The model under review builds one solid part; all positions refer to its coordinate system, in mm. A direction names the side the tool comes from. Round coordinates to 2 decimals unless told otherwise and drop trailing zeros. Write each loop counter-clockwise with the first axis right and the second up, starting at its lowest first coordinate (ties: lowest second). Pieces come first, ordered by that corner, then holes. Notation, with made-up numbers: (18, 17.5) -> (42, 17.5) arc R25 ccw to (42, 43.5) -> close; hole circle Ø5 at (5, 67.25). An arc over 180 degrees is marked (long way). Answer as a JSON object with one key per item and string values. Group by question number.
1) Machinability: for faces 5 (the flat face through (0, -20, 0)), 6 (the cylindrical face through (-50, -5, 0)), which of the approach directions +Z, -Z, +X, -X, +Y, -Y give a long, thin tool a straight path to every point of the face, cutting with its end or side? Answer none if there is none.
2) We need section B-B, the plane x = 0. Write out the cut boundary in (y, z), then the cut area to 3 significant figures.
3) We need section A-A, the plane y = -8.75. Write out the cut boundary in (x, z).
4) Mouldability with a two-part tool opening along X and no side actions: class faces 1 (the flat face through (23.664, -4.93, 14.526)), 2 (the flat face through (27, -10, 0)), 3 (the flat face through (-23.664, -4.93, -14.526)), 4 (the cylindrical face through (35, -5, 0)) as pulls with the +X half, pulls with the -X half, needs draft (parallel to the pull), parting line crosses it, or undercut.
5) To check wall thickness, follow probe 1 along Y at (x, z) = (-27, -7); probe 2 along Z at (x, y) = (40, -4); probe 3 along Z at (x, y) = (13.5, -26). State the ranges of each line that lie inside material, in increasing order. Write a range as [from, to].
6) We need section C-C, the plane x = -43. Write out the cut boundary in (y, z), then the cut area to 3 significant figures.
7) Insertion check: pin 1 Ø1 at (y, z) = (-15.5, -4.5) entering from -X; pin 2 Ø15 at (x, z) = (-5.5, -4.5) entering from -Y; pin 3 Ø3 at (x, z) = (-32.5, -7.5) entering from -Y; pin 4 Ø8 at (x, z) = (40, 0) entering from +Y. Each pin has a flat end and moves straight along its axis. Give the tip position at first contact, or say it passes through.
from build123d import *

# Parameters (mm, degrees)
F1_DEPTH = 10
F2_R     = 5
F3_DEPTH = 10.001
F5_DEPTH = 20
F6_R     = 15
F7_DEPTH = 10


with BuildPart() as f1:
    # F0 (on Front) → F1 (new body)
    with BuildSketch(Plane.XZ):
        with BuildLine():
            Line((5.158226, -19.323372), (41.659475, -9.861346))
            ThreePointArc((41.659475, -9.861346), (50, 0), (41.659475, 9.861346))
            Line((41.659475, 9.861346), (5.158226, 19.323372))
            ThreePointArc((5.158226, 19.323372), (15.861345, 12.182682), (20, 0))
            ThreePointArc((20, 0), (15.861345, -12.182682), (5.158226, -19.323372))
        make_face()
        with BuildLine():
            ThreePointArc((-5.158226, -19.323372), (0, -20), (5.158226, -19.323372))
            ThreePointArc((5.158226, -19.323372), (15.861345, -12.182682), (20, 0))
            ThreePointArc((20, 0), (15.861345, 12.182682), (5.158226, 19.323372))
            ThreePointArc((5.158226, 19.323372), (0, 20), (-5.158226, 19.323372))
            ThreePointArc((-5.158226, 19.323372), (-20, 0), (-5.158226, -19.323372))
        make_face()
        with BuildLine():
            Line((-41.659475, -9.861346), (-5.158226, -19.323372))
            ThreePointArc((-5.158226, -19.323372), (-20, 0), (-5.158226, 19.323372))
            Line((-5.158226, 19.323372), (-41.659475, 9.861346))
            ThreePointArc((-41.659475, 9.861346), (-50, 0), (-41.659475, -9.861346))
        make_face()
    extrude(amount=F1_DEPTH)

    # F2 (on face) → F3 (cut, through all)
    with BuildSketch(Plane.XZ.offset(10)):
        with Locations((40, 0)):
            Circle(F2_R)
        with Locations((-40, 0)):
            Circle(F2_R)
    extrude(amount=-F3_DEPTH, mode=Mode.SUBTRACT)

    # F4 (on face) → F5 (join)
    with BuildSketch(Plane.XZ.offset(10)):
        with BuildLine():
            ThreePointArc((5.158226, -19.323372), (15.861345, -12.182682), (20, 0))
            ThreePointArc((20, 0), (15.861345, 12.182682), (5.158226, 19.323372))
            ThreePointArc((5.158226, 19.323372), (0, 20), (-5.158226, 19.323372))
            ThreePointArc((-5.158226, 19.323372), (-20, 0), (-5.158226, -19.323372))
            ThreePointArc((-5.158226, -19.323372), (0, -20), (5.158226, -19.323372))
        make_face()
    extrude(amount=F5_DEPTH)

    # F6 (on face) → F7 (cut)
    with BuildSketch(Plane.XZ.offset(30)):
        Circle(F6_R)
    extrude(amount=-F7_DEPTH, mode=Mode.SUBTRACT)


solid = f1.part
Here are the results:
{
 "1": {"face 5": "-Y", "face 6": "-X, +Y, -Y"},
 "2": {"outline": "(-30, -20) -> (0, -20) -> (0, 20) -> (-30, 20) -> (-30, 15) -> (-20, 15) -> (-20, -15) -> (-30, -15) -> close", "area": "900 mm^2"},
 "3": {"outline": "(-41.66, -9.86) -> (-5.16, -19.32) arc R20 ccw to (5.16, -19.32) -> (41.66, -9.86) arc R10 ccw to (41.66, 9.86) -> (5.16, 19.32) arc R20 ccw to (-5.16, 19.32) -> (-41.66, 9.86) arc R10 ccw to start; hole circle Ø10 at (-40, 0); hole circle Ø10 at (40, 0)"},
 "4": {"face 1": "pulls with the +X half", "face 2": "needs draft", "face 3": "pulls with the -X half", "face 4": "undercut"},
 "5": {"probe 1": "y = [-10, 0]", "probe 2": "z = [-10.29, -5], [5, 10.29]", "probe 3": "z = [-14.76, -6.54], [6.54, 14.76]"},
 "6": {"outline": "(-10, -9.54) -> (0, -9.54) -> (0, -4) -> (-10, -4) -> close; (-10, 4) -> (0, 4) -> (0, 9.54) -> (-10, 9.54) -> close", "area": "111 mm^2"},
 "7": {"pin 1": "stops at x = -19.6", "pin 2": "stops at y = -20", "pin 3": "stops at y = -10", "pin 4": "passes through"}
}
